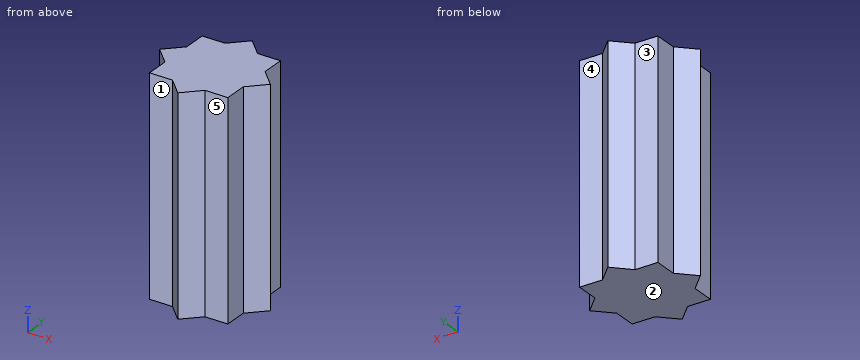
```python
from build123d import *

# Parameters (mm, degrees)
BOSS_EXTRUDE1_DEPTH      = 7.5
BOSS_EXTRUDE1_DEPTH_BACK = 7.5


with BuildPart() as part:
    # Sketch1 → Boss-Extrude1 (new, two sides: drawn at the far end of the back side and taken through both)
    with BuildSketch(Plane.XY.offset(-BOSS_EXTRUDE1_DEPTH_BACK)):
        Polygon((0, 3.9), (1.142283553, 2.757716447), (2.757716447, 2.757716447), (2.757716447, 1.142283553), (3.9, 0), (2.757716447, -1.142283553), (2.757716447, -2.757716447), (1.142283553, -2.757716447), (0, -3.9), (-1.142283553, -2.757716447), (-2.757716447, -2.757716447), (-2.757716447, -1.142283553), (-3.9, 0), (-2.757716447, 1.142283553), (-2.757716447, 2.757716447), (-1.142283553, 2.757716447), align=None)
    extrude(amount=BOSS_EXTRUDE1_DEPTH + BOSS_EXTRUDE1_DEPTH_BACK)


solid = part.part
```
Geometry: final body of the model. Coordinates: model frame, mm. Face numbers are marked on the shaded views. A direction names the side the tool comes from. Coordinates: 2 decimals unless noted, no trailing zeros. Loops run counter-clockwise (first coordinate to the right, second up) from the corner with the lowest first, then second, coordinate; pieces in that order, holes last. Notation, with made-up numbers: M 84.5,37.25 L 92.5,37.25 A14 cw 92.5,63.25 Z; hole C 14.25,2.5 d4. An arc over 180 degrees is marked long. Put each result on its own line as item: value.
(1) Material intervals for probe 1 along Y at (x, z) = (-1.75, 4); probe 2 along X at (y, z) = (-3, -1.5), sorted ascending.
Answer sheet:
probe 1: y = -2.76 to 2.76
probe 2: x = -0.9 to 0.9
(2) Cut plane C-C on y = -3.5. Return the cut outline in (x, z), then the cut area to 3 significant figures.
Answer sheet:
outline: M -0.4,-7.5 L 0.4,-7.5 L 0.4,7.5 L -0.4,7.5 Z
area: 12.0 mm^2
(3) Access query for the marked faces 1, 2, 3, 4 and 5. Directions: +Z, -Z, +X, -X, +Y, -Y. A direction counts if a zero-diameter tool reaches every point of the face in a straight line with its end or side. Return the directions, or none.
Answer sheet:
face 1: +Z, -Z, -X, -Y
face 2: -Z, +X, -X, +Y, -Y
face 3: +Z, -Z, -X, +Y
face 4: +Z, -Z, +X, +Y
face 5: +Z, -Z, +X, -Y
(4) Cut plane A-A on z = -3.75. Return the cut outline in (x, y).
Answer sheet:
outline: M -3.9,0 L -2.76,-1.14 L -2.76,-2.76 L -1.14,-2.76 L 0,-3.9 L 1.14,-2.76 L 2.76,-2.76 L 2.76,-1.14 L 3.9,0 L 2.76,1.14 L 2.76,2.76 L 1.14,2.76 L 0,3.9 L -1.14,2.76 L -2.76,2.76 L -2.76,1.14 Z
(5) Cut plane B-B on x = -3. Return the cut outline in (y, z), then the cut area to 3 significant figures.
Answer sheet:
outline: M -0.9,-7.5 L 0.9,-7.5 L 0.9,7.5 L -0.9,7.5 Z
area: 27.0 mm^2
(6) First-contact query: pin 1 (1.3 mm diameter, centred on y = 2, z = -0.5, fed in from -X); pin 2 (1.5 mm diameter, centred on x = -1.5, z = -2.5, fed in from +Y); pin 3 (0.8 mm diameter, centred on x = -2, z = 0.5, fed in from +Y). Flat tips, straight axial feed; report the tip coordinate or a pass-through.
Answer sheet:
pin 1: stops at x = -2.76
pin 2: stops at y = 3.15
pin 3: stops at y = 2.76
